Autodesk Inventor part; units mm, degrees
ref_plane "YZ Plane" through (0, 0, 0) normal (1, 0, 0) x (0, 1, 0)
ref_plane "XZ Plane" through (0, 0, 0) normal (0, 1, 0) x (-1, 0, 0)
ref_plane "XY Plane" through (0, 0, 0) normal (0, 0, 1) x (1, 0, 0)
sketch "Sketch1" plane through (0, 0, 0) normal (0, 0, 1) x (1, 0, 0)
  line L0 (6.35, 3.6662) -> (6.35, -3.6662)
  line L1 (6.35, -3.6662) -> (0, -7.3323)
  line L2 (0, -7.3323) -> (-6.35, -3.6662)
  line L3 (-6.35, -3.6662) -> (-6.35, 3.6662)
  line L4 (-6.35, 3.6662) -> (0, 7.3323)
  line L5 (0, 7.3323) -> (6.35, 3.6662)
  point P0 (0, 0)
  point P1 (0, 0)
  dimension "d0" = 12.7
extrude "Extrusion1" add sketch "Sketch1" along normal blind 71
sketch "Sketch2" plane through (0, 0, 0) normal (0, 1, 0) x (-1, 0, 0)
  line L0 (15, 67.5) -> (5, 67.5)
  line L1 (5, 67.5) -> (5, 69)
  line L2 (5, 69) -> (15, 69)
  line L3 (15, 69) -> (15, 67.5)
  line L4 (15, 22.5) -> (5, 22.5)
  line L5 (5, 22.5) -> (5, 24)
  line L6 (5, 24) -> (15, 24)
  line L7 (15, 24) -> (15, 22.5)
  line L8 (15, 1.5) -> (5, 1.5)
  line L9 (5, 1.5) -> (5, 3)
  line L10 (5, 3) -> (15, 3)
  line L11 (15, 3) -> (15, 1.5)
  line L12 (0, 71) -> (6.35, 71)
  line L13 (0, 0) -> (0, 71)
  line L14 (0, -14) -> (0, 84)
  dimension "d3" = 2
  dimension "d4" = 1.5
  dimension "d5" = 47
  dimension "d6" = 68
  dimension "d7" = 10
  dimension "d8" = 5
revolve "Revolution1" cut sketch "Sketch2" angle 360 about axis through (0, 0, -10) along (0, 0, 1)
properties part number "Performance Axle"
Can you work these out from the model? Positions are in its coordinate system, mm. A direction names the side the tool comes from. Give positions to 0.01 mm unless a question says otherwise; leave off trailing zeros. Loops run counter-clockwise (first coordinate to the right, second up) from the corner with the lowest first, then second, coordinate; pieces in that order, holes last. Notation, with made-up numbers: (53.25, 77.25) - (62.25, 77.25) arc R23 ccw to (62.25, 93.25) - close; hole circle Ø8 at (-6, 33.5). An arc over 180 degrees is marked (long way). One line per item, written item: value.
(1) I need wall thicknesses on line 1 along Z through (x, y) = (5.5, -2.5); line 2 along Y through (x, z) = (1, 10); line 3 along Y through (x, z) = (-0.5, 35). Which ranges of each line are inside material? Lowest first, please.
Verdict:
line 1: 0 to 1.5, 3 to 22.5, 24 to 67.5, 69 to 71
line 2: -6.75 to 6.75
line 3: -7.04 to 7.04
(2) On a 3-axis mill with a long thin cutter (end or side, diameter ignored), from which of +Z, -Z, +X, -X, +Y, -Y can I reach the whole of each face in a straight line? I mean faces 1 (the face through (1.08, 4.88, 2.26)), 2 (the face through (6.35, 0, 45)). Say none if no direction works.
Verdict:
face 1: none
face 2: +Z, -Z, +X, +Y, -Y
(3) If we section it at C-C, the plane z = 45.5: List the corners of the cut face in (x, y) for me, plus the area to 3 significant figures.
Verdict:
outline: (-6.35, -3.67) - (0, -7.33) - (6.35, -3.67) - (6.35, 3.67) - (0, 7.33) - (-6.35, 3.67) - close
area: 140 mm^2
(4) If we section it at A-A, the plane y = 6: List the corners of the cut face in (x, z) for me, plus the area to 3 significant figures.
Verdict:
outline: (-2.31, 0) - (2.31, 0) - (2.31, 1.5) - (-2.31, 1.5) - close; (-2.31, 3) - (2.31, 3) - (2.31, 22.5) - (-2.31, 22.5) - close; (-2.31, 24) - (2.31, 24) - (2.31, 67.5) - (-2.31, 67.5) - close; (-2.31, 69) - (2.31, 69) - (2.31, 71) - (-2.31, 71) - close
area: 307 mm^2
(5) If we section it at D-D, the plane x = 3.25: List the corners of the cut face in (y, z) for me, plus the area to 3 significant figures.
Verdict:
outline: (-5.46, 0) - (5.46, 0) - (5.46, 1.5) - (3.8, 1.5) - (3.8, 3) - (5.46, 3) - (5.46, 22.5) - (3.8, 22.5) - (3.8, 24) - (5.46, 24) - (5.46, 67.5) - (3.8, 67.5) - (3.8, 69) - (5.46, 69) - (5.46, 71) - (-5.46, 71) - (-5.46, 69) - (-3.8, 69) - (-3.8, 67.5) - (-5.46, 67.5) - (-5.46, 24) - (-3.8, 24) - (-3.8, 22.5) - (-5.46, 22.5) - (-5.46, 3) - (-3.8, 3) - (-3.8, 1.5) - (-5.46, 1.5) - close
area: 760 mm^2
(6) If we mould it in two halves opening along Z, with no side actions, what happens to faces 3 (the face through (-3.131, -5.525, 0.74)), 4 (the face through (0, 0, 71)), 5 (the face through (5, -2, 3))? For each: released by +Z, released by -Z, zero draft, split by the parting line, or undercut.
Verdict:
face 3: zero draft
face 4: released by +Z
face 5: undercut
(7) If we section it at B-B, the plane y = 1.5: List the corners of the cut face in (x, z) for me, plus the area to 3 significant figures.
Verdict:
outline: (-6.35, 0) - (6.35, 0) - (6.35, 1.5) - (4.77, 1.5) - (4.77, 3) - (6.35, 3) - (6.35, 22.5) - (4.77, 22.5) - (4.77, 24) - (6.35, 24) - (6.35, 67.5) - (4.77, 67.5) - (4.77, 69) - (6.35, 69) - (6.35, 71) - (-6.35, 71) - (-6.35, 69) - (-4.77, 69) - (-4.77, 67.5) - (-6.35, 67.5) - (-6.35, 24) - (-4.77, 24) - (-4.77, 22.5) - (-6.35, 22.5) - (-6.35, 3) - (-4.77, 3) - (-4.77, 1.5) - (-6.35, 1.5) - close
area: 887 mm^2
